Check sheet for the drawn part. Datum: minimum x, y, z corner. Units: mm. Round coordinates to 2 decimals unless told otherwise and drop trailing zeros. Order: outer loops, then holes, each group sorted by start corner. A loop starts at its lowest first (then second) coordinate and runs counter-clockwise, first axis right, second up.
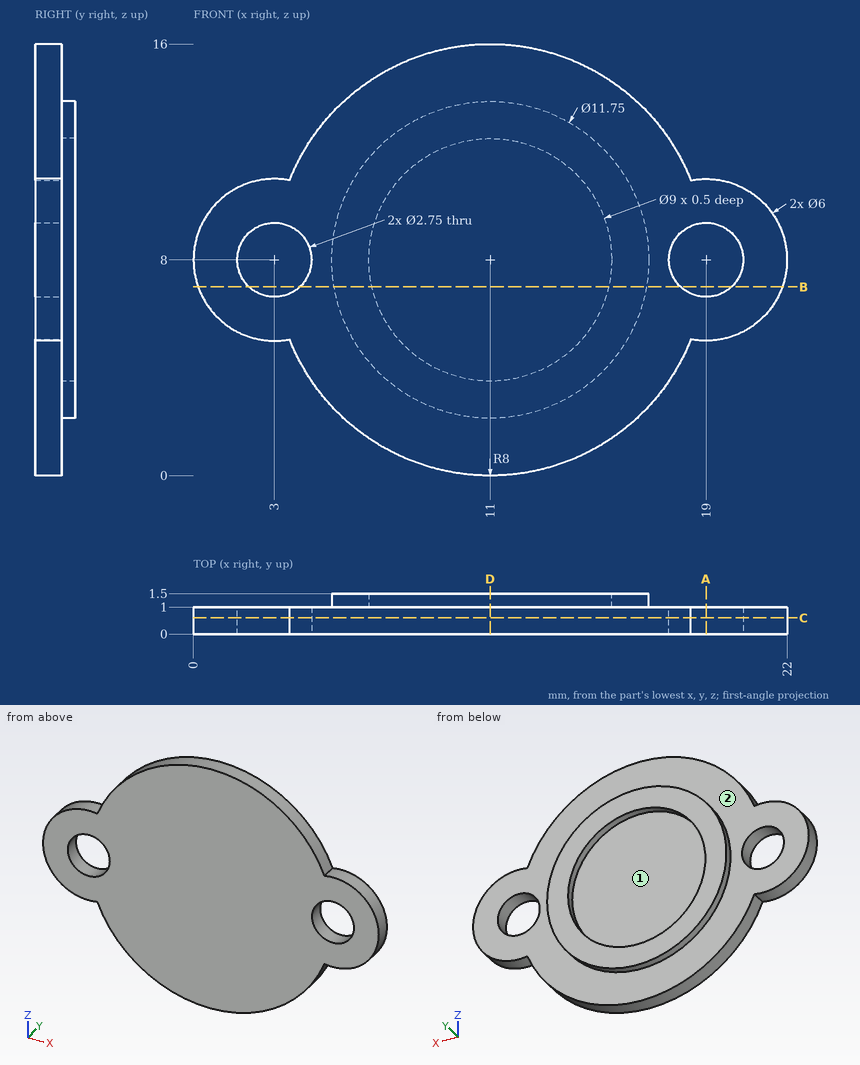
(1) Sectioned sample at C-C, the plane y = 0.6. Give the number of separate pieces and of enclosed holes in the cut face, and give its area (3 significant figures).
Returned:
separate pieces: 1
enclosed holes: 2
area: 220 mm2
(2) Sectioned sample at A-A, the plane x = 19. Record the cut outline in (y, z) (3 decimals).
Returned:
outline: (0, 5) - (1, 5) - (1, 6.625) - (0, 6.625) - close; (0, 9.375) - (1, 9.375) - (1, 11) - (0, 11) - close
(3) Sectioned sample at D-D, the plane x = 11. Record the cut outline in (y, z) (3 decimals).
Returned:
outline: (0, 0) - (1, 0) - (1, 2.125) - (1.5, 2.125) - (1.5, 3.5) - (1, 3.5) - (1, 12.5) - (1.5, 12.5) - (1.5, 13.875) - (1, 13.875) - (1, 16) - (0, 16) - close
(4) Sectioned sample at B-B, the plane z = 7. Record the cut outline in (x, y), and give its area (3 significant figures).
Returned:
outline: (0.17, 0) - (2.06, 0) - (2.06, 1) - (0.17, 1) - close; (3.94, 0) - (18.06, 0) - (18.06, 1) - (16.79, 1) - (16.79, 1.5) - (15.39, 1.5) - (15.39, 1) - (6.61, 1) - (6.61, 1.5) - (5.21, 1.5) - (5.21, 1) - (3.94, 1) - close; (19.94, 0) - (21.83, 0) - (21.83, 1) - (19.94, 1) - close
area: 19.3 mm2
(5) Draft check along Z on the marked faces 1 and 2. Enter one of: released by +Z, released by -Z, zero draft, split by the parting line, or undercut.
Returned:
face 1: undercut
face 2: zero draft
(6) Material ranges on line 1 (X direction, y = 1.3, z = 8) (3 decimals); line 2 (Z direction, x = 3, y = 0.3) (3 decimals); line 3 (X direction, y = 0.7, z = 9), recorded low to high.
Returned:
line 1: x = 5.125 to 6.5, 15.5 to 16.875
line 2: z = 5 to 6.625, 9.375 to 11
line 3: x = 0.17 to 2.06, 3.94 to 18.06, 19.94 to 21.83
(7) Depth check by flat-ended pin: P1, Ø6, axis at x = 3, z = 14.5, coming from the +Y side. Enter the tip coordinate at first touch or a pass-through.
Returned:
P1: stops at y = 1
